Can you work these out from the model? Positions are in its coordinate system, mm. A direction names the side the tool comes from. Give positions to 0.01 mm unless a question says otherwise; leave off trailing zeros. Order: outer loops, then holes, each group sorted by start corner. A loop starts at its lowest first (then second) coordinate and runs counter-clockwise, first axis right, second up.
```python
from build123d import *

# Parameters (mm, degrees)
SKETCH1_W          = 101.6
SKETCH1_H          = 101.6
SKETCH1_W_2        = 76.2
SKETCH1_H_2        = 76.2
EXTRUDE1_DEPTH     = 304.8
FILLET1_R          = 3.175
SKETCH2_R          = 22.225
CUT_EXTRUDE1_DEPTH = 326.278711262
SKETCH3_R          = 12.7
EXTRUDE2_DEPTH     = 12.7
SKETCH6_R          = 12.7
EXTRUDE3_DEPTH     = 12.7
SKETCH7_R          = 22.225
CUT_EXTRUDE2_DEPTH = 427.633056619
FILLET2_R          = 12.7


with BuildPart() as part:
    # Sketch1 → Extrude1 (new body)
    with BuildSketch(Plane.XY):
        Rectangle(SKETCH1_W, SKETCH1_H)
        Rectangle(SKETCH1_W_2, SKETCH1_H_2, mode=Mode.SUBTRACT)
    extrude(amount=EXTRUDE1_DEPTH)

    # Fillet1
    fillet1_edges = [part.edges().sort_by_distance(p)[0] for p in [
        (-38.1, 38.1, 152.4),
        (-38.1, -38.1, 152.4),
        (38.1, -38.1, 152.4),
        (38.1, 38.1, 152.4),
        (-50.8, 50.8, 152.4),
        (50.8, 50.8, 152.4),
        (50.8, -50.8, 152.4),
        (-50.8, -50.8, 152.4),
    ]]
    fillet(fillet1_edges, radius=FILLET1_R)

    # Sketch2 → Cut-Extrude1 (cut, through all)
    with BuildSketch(Plane(origin=(50.8, 0, 0), x_dir=(0, 0, -1), z_dir=(1, 0, 0))):
        with Locations((-44.45, 0)):
            Circle(SKETCH2_R)
    extrude(amount=-CUT_EXTRUDE1_DEPTH, mode=Mode.SUBTRACT)

    # Sketch3 → Extrude2 (add, symmetric)
    with BuildSketch(Plane(origin=(0, 0, 0), x_dir=(1, 0, 0), z_dir=(0, 1, 0))):
        with BuildLine():
            Line((-50.8, -304.8), (-69.85, -304.8))
            Line((-69.85, -304.8), (-88.9, -260.35))
            Line((-88.9, -260.35), (-127, -260.35))
            ThreePointArc((-127, -260.35), (-162.440231571, -271.420694713), (-184.15, -241.3))
            Line((-184.15, -241.3), (-184.15, -114.3))
            Line((-184.15, -114.3), (-50.8, -114.3))
            Line((-50.8, -114.3), (-50.8, -304.8))
        make_face()
        with Locations(Location((-152.4, -241.3, 0), (0, 0, 270))):
            Circle(SKETCH3_R, mode=Mode.SUBTRACT)
    extrude(amount=EXTRUDE2_DEPTH, both=True)

    # Sketch6 → Extrude3 (add, symmetric)
    with BuildSketch(Plane(origin=(0, 0, 0), x_dir=(0, 0, -1), z_dir=(1, 0, 0))):
        with BuildLine():
            Line((-190.5, -50.8), (-190.5, -184.15))
            Line((-190.5, -184.15), (-63.5, -184.15))
            ThreePointArc((-63.5, -184.15), (-33.379305287, -162.440231571), (-44.45, -127))
            Line((-44.45, -127), (-44.45, -88.9))
            Line((-44.45, -88.9), (0, -69.85))
            Line((0, -69.85), (0, -50.8))
            Line((0, -50.8), (-190.5, -50.8))
        make_face()
        with Locations((-63.5, -152.4)):
            Circle(SKETCH6_R, mode=Mode.SUBTRACT)
    extrude(amount=EXTRUDE3_DEPTH, both=True)

    # Sketch7 → Cut-Extrude2 (cut, through all)
    with BuildSketch(Plane(origin=(0, 50.8, 0), x_dir=(-1, 0, 0), z_dir=(0, 1, 0))):
        with Locations(Location((0, 254, 0), (0, 0, 90))):
            Circle(SKETCH7_R)
    extrude(amount=-CUT_EXTRUDE2_DEPTH, mode=Mode.SUBTRACT)

    # Fillet2
    fillet2_edges = [part.edges().sort_by_distance(p)[0] for p in [
        (12.7, -50.8, 95.25),
        (-12.7, -50.8, 95.25),
        (0, -50.8, 190.5),
        (-50.8, 12.7, 209.55),
        (-50.8, -12.7, 209.55),
        (-50.8, 0, 114.3),
    ]]
    fillet(fillet2_edges, radius=FILLET2_R)


solid = part.part
```
1) If I drill on line 1 (Y direction, x = 3, z = 63); line 2 (Y direction, x = 0.25, z = 63.5); line 3 (X direction, y = -24, z = 40), over which ranges is the centre line in solid material (lowest first)?
2) Which directions (+Z, -Z, +X, -X, +Y, -Y) give clear straight access to the entire face, cutting with the end or side of a thin tool? Please do faces 1 (the face through (-79.24, 0.18, 282.89)), 2 (the face through (-50.8, -32, 116)), 3 (the face through (-123, 12.7, 187)).
3) Suppose I cut it at A-A (x = 0). Please give me the cut outline in (y, z) (3 decimals).
4) I'm going to push flat-ended pins straight in: pin 1 Ø3 at (x, y) = (-74.5, 12) entering from +Z; pin 2 Ø7.5 at (x, y) = (-3.5, -107.5) entering from +Z; pin 3 Ø7.5 at (x, y) = (-131.5, 0) entering from -Z; pin 4 Ø15 at (x, z) = (-152.4, 241.3) entering from -Y. Where does each tip first touch, or does it pass through?
5) Suppose I cut it at B-B (y = -152.4). Please give me the cut outline in (x, z), and give its area (3 significant figures).
6) Suppose I cut it at C-C (x = -152.4). Please give me the cut outline in (y, z).
7) We'd pull the mould along Y, two halves only. Please class faces 4 (the face through (-0.36, -53.02, 196.03)), 5 (the face through (-38.1, 0, 150)), 6 (the face through (12.7, -123, 118)): +Y half, -Y half, draft (parallel to the pull), parting line (faces both ways), or undercut.
8) Suppose I cut it at D-D (z = 161.5). Please give me the cut outline in (x, y) (3 decimals), and give its area (3 significant figures).
Results:
1. line 1: y = -184.15 to -165.09, -139.71 to -38.1, 38.1 to 50.8
1. line 2: y = -184.15 to -165.1, -139.7 to -38.1, 38.1 to 50.8
1. line 3: x = -50.8 to -38.1, 38.1 to 50.8
2. face 1: +Z, +Y, -Y
2. face 2: -Z, -X
2. face 3: +Z, -Z, -X, +Y
3. outline: (-184.15, 63.5) arc R31.75 ccw to (-127, 44.45) - (-88.9, 44.45) - (-69.85, 0) - (-38.1, 0) - (-38.1, 231.775) - (-50.8, 231.775) - (-50.8, 203.2) arc R12.7 cw to (-63.5, 190.5) - (-184.15, 190.5) - close; (-50.8, 276.225) - (-38.1, 276.225) - (-38.1, 304.8) - (-50.8, 304.8) - close; (38.1, 0) - (50.8, 0) - (50.8, 231.775) - (38.1, 231.775) - close; (38.1, 276.225) - (50.8, 276.225) - (50.8, 304.8) - (38.1, 304.8) - close; hole circle Ø25.4 at (-152.4, 63.5)
4. pin 1: stops at z = 297.45
4. pin 2: stops at z = 190.5
4. pin 3: stops at z = 114.3
4. pin 4: passes through
5. outline: (-12.7, 31.75) - (12.7, 31.75) - (12.7, 50.8) - (-12.7, 50.8) - close; (-12.7, 76.2) - (12.7, 76.2) - (12.7, 190.5) - (-12.7, 190.5) - close
5. area: 3,390 mm2
6. outline: (-12.7, 114.3) - (12.7, 114.3) - (12.7, 228.6) - (-12.7, 228.6) - close; (-12.7, 254) - (12.7, 254) - (12.7, 273.05) - (-12.7, 273.05) - close
7. face 4: -Y half
7. face 5: undercut
7. face 6: draft
8. outline: (-184.15, -12.7) - (-63.5, -12.7) arc R12.7 cw to (-50.8, -25.4) - (-50.8, -47.625) arc R3.175 ccw to (-47.625, -50.8) - (-25.4, -50.8) arc R12.7 cw to (-12.7, -63.5) - (-12.7, -184.15) - (12.7, -184.15) - (12.7, -63.5) arc R12.7 cw to (25.4, -50.8) - (47.625, -50.8) arc R3.175 ccw to (50.8, -47.625) - (50.8, 47.625) arc R3.175 ccw to (47.625, 50.8) - (-47.625, 50.8) arc R3.175 ccw to (-50.8, 47.625) - (-50.8, 25.4) arc R12.7 cw to (-63.5, 12.7) - (-184.15, 12.7) - close; hole (-38.1, -34.925) arc R3.175 ccw to (-34.925, -38.1) - (34.925, -38.1) arc R3.175 ccw to (38.1, -34.925) - (38.1, 34.925) arc R3.175 ccw to (34.925, 38.1) - (-34.925, 38.1) arc R3.175 ccw to (-38.1, 34.925) - close
8. area: 11,400 mm2
